The figure shows three views and two pictorial views of one solid part (mm, origin at its lowest corner). Answer the questions. A direction names the side the tool comes from. Give positions to 0.01 mm unless a question says otherwise; leave off trailing zeros. Order: outer loops, then holes, each group sorted by start corner. A loop starts at its lowest first (then second) coordinate and runs counter-clockwise, first axis right, second up. Notation, with made-up numbers: (-12.5, 6) - (13.5, 6) arc R20 cw to (13.5, 23) - close; hole circle Ø11 at (86, 13). An arc over 180 degrees is marked (long way). Answer as CSV lines item,"result". Start each with the question number.
1. Section B-B on y = 3 is taken. Give the vertices of the cut face in (x, z) (1 decimal), and give its area (3 significant figures).
2. Determine the mould class of the marked faces 6, 7, 8 and 9 for opening direction X: +X half, -X half, draft (parallel to the pull), parting line (faces both ways), or undercut.
3. Section C-C on x = 11 is taken. Give the vertices of the cut face in (y, z).
4. Consider line 1 along X through (y, z) = (1.5, 16) (1 decimal); line 2 along Z through (x, y) = (7.5, 2.5); line 3 along Z through (x, y) = (15, 10.5) (1 decimal). Determine where each line is inside the solid, lowest interval first. Write a range as [from, to].
5. Flat-ended cylindrical pins translate along their axes: pin 1 (7 mm diameter, centred on x = 4, z = 21, fed in from +Y); pin 2 (3 mm diameter, centred on x = 8.5, y = 2.5, fed in from -Z); pin 3 (7 mm diameter, centred on x = 6, y = 2.5, fed in from +Z); pin 4 (2 mm diameter, centred on y = 10.414, z = 5.588, fed in from +X). Find the tip coordinate at first contact, or state that the pin passes through.
6. Section D-D on z = 14 is taken. Give the vertices of the cut face in (x, y) (1 decimal).
7. Section A-A on z = 22 is taken. Give the vertices of the cut face in (x, y) (1 decimal).
8. Which of the six approach directions +Z, -Z, +X, -X, +Y, -Y give full straight-line access (tool end or side, diameter ignored) to the marked faces 1, 2, 3, 4 and 5?
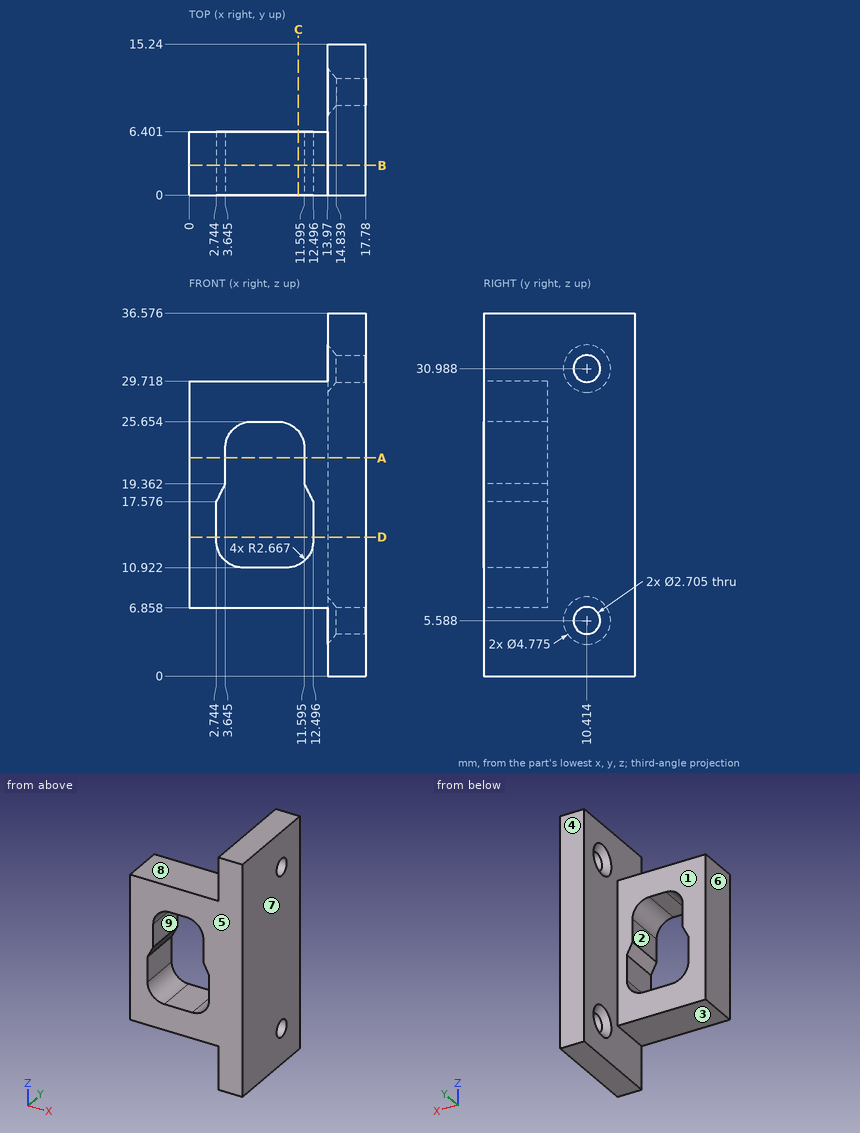
Checks:
1,outline,"(0, 6.9) - (14, 6.9) - (14, 0) - (17.8, 0) - (17.8, 36.6) - (14, 36.6) - (14, 29.7) - (0, 29.7) - close; hole (2.7, 13.6) arc R2.7 ccw to (5.4, 10.9) - (9.8, 10.9) arc R2.7 ccw to (12.5, 13.6) - (12.5, 17.6) - (11.6, 19.4) - (11.6, 23) arc R2.7 ccw to (8.9, 25.7) - (6.3, 25.7) arc R2.7 ccw to (3.6, 23) - (3.6, 19.4) - (2.7, 17.6) - close"
1,area,"334 mm²"
2,face 6,"-X half"
2,face 7,"+X half"
2,face 8,"draft"
2,face 9,"undercut"
3,outline,"(0, 6.86) - (6.4, 6.86) - (6.4, 11.19) - (0, 11.19) - close; (0, 24.67) - (6.4, 24.67) - (6.4, 29.72) - (0, 29.72) - close"
4,line 1,"x = [0, 2.7], [12.5, 17.8]"
4,line 2,"z = [6.86, 10.92], [25.65, 29.72]"
4,line 3,"z = [0, 4.2], [6.9, 29.6], [32.3, 36.6]"
5,pin 1,"stops at y = 6.4"
5,pin 2,"stops at z = 6.86"
5,pin 3,"stops at z = 29.72"
5,pin 4,"passes through"
6,outline,"(0, 0) - (2.7, 0) - (2.7, 6.4) - (0, 6.4) - close; (12.5, 0) - (17.8, 0) - (17.8, 15.2) - (14, 15.2) - (14, 6.4) - (12.5, 6.4) - close"
7,outline,"(0, 0) - (3.6, 0) - (3.6, 6.4) - (0, 6.4) - close; (11.6, 0) - (17.8, 0) - (17.8, 15.2) - (14, 15.2) - (14, 6.4) - (11.6, 6.4) - close"
8,face 1,"+Z, -Z, -X, +Y"
8,face 2,"+Y, -Y"
8,face 3,"-Z, -X, +Y, -Y"
8,face 4,"+Z, -Z, +X, -X, +Y"
8,face 5,"+Z, -Z, +X, -X, -Y"
